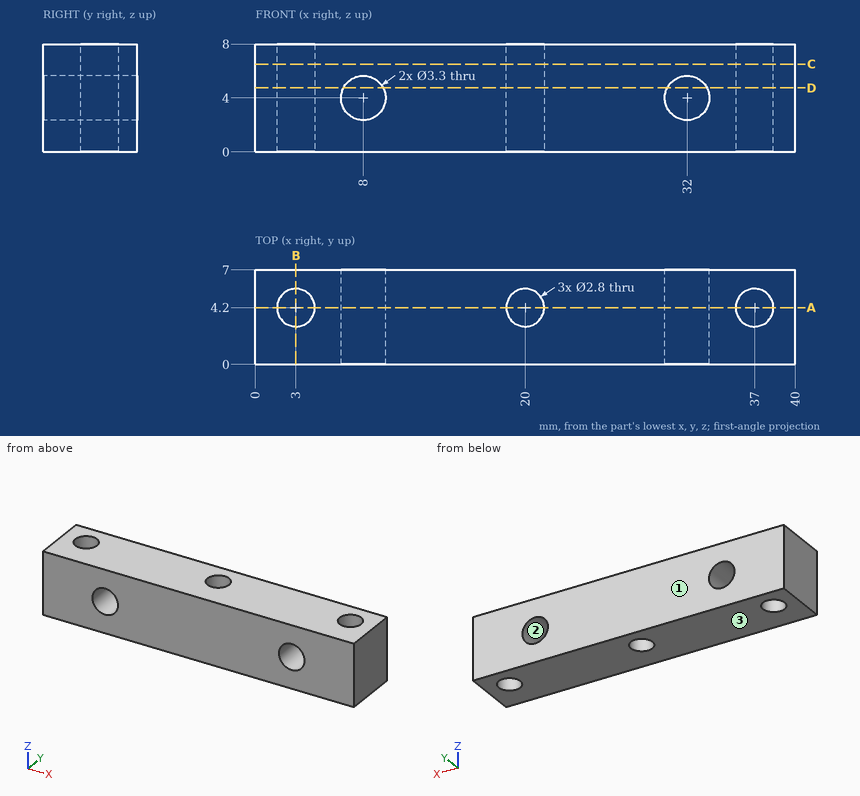
Here's the drawing with two shaded views (mm, measured from the low corner). I have some questions. Coordinates: 2 decimals unless noted, no trailing zeros. Write each loop counter-clockwise with the first axis right and the second up, starting at its lowest first coordinate (ties: lowest second). Pieces come first, ordered by that corner, then holes. Notation, with made-up numbers: (46, 60.25) - (86, 60.25) arc R27 ccw to (86, 92.25) - close; hole circle Ø6 at (57.5, 12.25). An arc over 180 degrees is marked (long way). Return JSON: item names as keys, results as strings.
Q1. Please list where these lines run through material, in increasing order: L1, parallel to Y at x = 37, z = 6.25; L2, parallel to Z at x = 32, y = 5.5; L3, parallel to X at y = 6.25, z = 3.5. Write a range as from..to.
Computed values:
{"L1": "y = 0..2.8, 5.6..7", "L2": "z = 0..2.35, 5.65..8", "L3": "x = 0..6.43, 9.57..30.43, 33.57..40"}
Q2. I'm going to push flat-ended pins straight in: pin 1 Ø3 at (x, y) = (3, 4.2) entering from -Z; pin 2 Ø3 at (x, z) = (32, 4) entering from +Y. Where does each tip first touch, or does it pass through?
Computed values:
{"pin 1": "stops at z = 0", "pin 2": "passes through"}
Q3. Thinking about a two-plate mould opening in Z: for the marked faces 1, 2 and 3, which applies, +Z half, -Z half, draft (parallel to the pull), parting line (faces both ways), or undercut?
Computed values:
{"face 1": "draft", "face 2": "undercut", "face 3": "-Z half"}
Q4. If we section it at A-A (y = 4.2): Please give me the cut outline in (x, z), then the cut area to 3 significant figures.
Computed values:
{"outline": "(0, 0) - (1.6, 0) - (1.6, 8) - (0, 8) - close; (4.4, 0) - (18.6, 0) - (18.6, 8) - (4.4, 8) - close; (21.4, 0) - (35.6, 0) - (35.6, 8) - (21.4, 8) - close; (38.4, 0) - (40, 0) - (40, 8) - (38.4, 8) - close; hole circle Ø3.3 at (8, 4); hole circle Ø3.3 at (32, 4)", "area": "236 mm2"}
Q5. If we section it at D-D (z = 4.75): Please give me the cut outline in (x, y), then the cut area to 3 significant figures.
Computed values:
{"outline": "(0, 0) - (6.53, 0) - (6.53, 7) - (0, 7) - close; (9.47, 0) - (30.53, 0) - (30.53, 7) - (9.47, 7) - close; (33.47, 0) - (40, 0) - (40, 7) - (33.47, 7) - close; hole circle Ø2.8 at (3, 4.2); hole circle Ø2.8 at (20, 4.2); hole circle Ø2.8 at (37, 4.2)", "area": "220 mm2"}
Q6. If we section it at C-C (z = 6.5): Please give me the cut outline in (x, y), then the cut area to 3 significant figures.
Computed values:
{"outline": "(0, 0) - (40, 0) - (40, 7) - (0, 7) - close; hole circle Ø2.8 at (3, 4.2); hole circle Ø2.8 at (20, 4.2); hole circle Ø2.8 at (37, 4.2)", "area": "262 mm2"}
Q7. If we section it at B-B (x = 3): Please give me the cut outline in (y, z).
Computed values:
{"outline": "(0, 0) - (2.8, 0) - (2.8, 8) - (0, 8) - close; (5.6, 0) - (7, 0) - (7, 8) - (5.6, 8) - close"}
